from build123d import *

# Parameters (mm, degrees)
SKETCH1_R           = 14.2875
BOSS_EXTRUDE1_DEPTH = 3.175
CUT_EXTRUDE1_REACH  = 5.175
SKETCH2_R           = 2.667
CUT_EXTRUDE2_REACH  = 5.175
SKETCH4_R           = 6.35


with BuildPart() as part:
    # Sketch1 → Boss-Extrude1 (new body)
    with BuildSketch(Plane(origin=(0, 0, 0), x_dir=(1, 0, 0), z_dir=(0, 1, 0))):
        with BuildLine():
            Line((0, 25.4), (203.2, 25.4))
            ThreePointArc((203.2, 25.4), (228.6, 0), (203.2, -25.4))
            Line((203.2, -25.4), (0, -25.4))
            ThreePointArc((0, -25.4), (-25.4, 0), (0, 25.4))
        make_face()
        Circle(SKETCH1_R, mode=Mode.SUBTRACT)
        with Locations((203.2, 0)):
            Circle(SKETCH1_R, mode=Mode.SUBTRACT)
    extrude(amount=BOSS_EXTRUDE1_DEPTH)

    # Sketch2 → Cut-Extrude1 (cut, up to next)
    with BuildSketch(Plane(origin=(0, 3.175, 0), x_dir=(1, 0, 0), z_dir=(0, 1, 0)), mode=Mode.PRIVATE) as cut_extrude1_sk1:
        with Locations((101.6, 0)):
            Circle(SKETCH2_R)
    cut_extrude1_tool1 = extrude(cut_extrude1_sk1.sketch, amount=-CUT_EXTRUDE1_REACH, mode=Mode.PRIVATE) & part.part
    add(cut_extrude1_tool1.solids().sort_by_distance((101.6, 3.175, 0))[0], mode=Mode.SUBTRACT)

    # Sketch4 → Cut-Extrude2 (cut, up to next)
    with BuildSketch(Plane.XZ, mode=Mode.PRIVATE) as cut_extrude2_sk1:
        with Locations((30.1625, -12.7)):
            Circle(SKETCH4_R)
    cut_extrude2_tool1 = extrude(cut_extrude2_sk1.sketch, amount=-CUT_EXTRUDE2_REACH, mode=Mode.PRIVATE) & part.part
    add(cut_extrude2_tool1.solids().sort_by_distance((30.1625, 0, -12.7))[0], mode=Mode.SUBTRACT)
    # Sketch4 → Cut-Extrude2 (cut, up to next)
    with BuildSketch(Plane.XZ, mode=Mode.PRIVATE) as cut_extrude2_sk2:
        with Locations((49.2125, -12.7)):
            Circle(SKETCH4_R)
    cut_extrude2_tool2 = extrude(cut_extrude2_sk2.sketch, amount=-CUT_EXTRUDE2_REACH, mode=Mode.PRIVATE) & part.part
    add(cut_extrude2_tool2.solids().sort_by_distance((49.2125, 0, -12.7))[0], mode=Mode.SUBTRACT)
    # Sketch4 → Cut-Extrude2 (cut, up to next)
    with BuildSketch(Plane.XZ, mode=Mode.PRIVATE) as cut_extrude2_sk3:
        with Locations((68.2625, -12.7)):
            Circle(SKETCH4_R)
    cut_extrude2_tool3 = extrude(cut_extrude2_sk3.sketch, amount=-CUT_EXTRUDE2_REACH, mode=Mode.PRIVATE) & part.part
    add(cut_extrude2_tool3.solids().sort_by_distance((68.2625, 0, -12.7))[0], mode=Mode.SUBTRACT)
    # Sketch4 → Cut-Extrude2 (cut, up to next)
    with BuildSketch(Plane.XZ, mode=Mode.PRIVATE) as cut_extrude2_sk4:
        with Locations((87.3125, -12.7)):
            Circle(SKETCH4_R)
    cut_extrude2_tool4 = extrude(cut_extrude2_sk4.sketch, amount=-CUT_EXTRUDE2_REACH, mode=Mode.PRIVATE) & part.part
    add(cut_extrude2_tool4.solids().sort_by_distance((87.3125, 0, -12.7))[0], mode=Mode.SUBTRACT)
    # Sketch4 → Cut-Extrude2 (cut, up to next)
    with BuildSketch(Plane.XZ, mode=Mode.PRIVATE) as cut_extrude2_sk5:
        with Locations((106.3625, -12.7)):
            Circle(SKETCH4_R)
    cut_extrude2_tool5 = extrude(cut_extrude2_sk5.sketch, amount=-CUT_EXTRUDE2_REACH, mode=Mode.PRIVATE) & part.part
    add(cut_extrude2_tool5.solids().sort_by_distance((106.3625, 0, -12.7))[0], mode=Mode.SUBTRACT)
    # Sketch4 → Cut-Extrude2 (cut, up to next)
    with BuildSketch(Plane.XZ, mode=Mode.PRIVATE) as cut_extrude2_sk6:
        with Locations((125.4125, -12.7)):
            Circle(SKETCH4_R)
    cut_extrude2_tool6 = extrude(cut_extrude2_sk6.sketch, amount=-CUT_EXTRUDE2_REACH, mode=Mode.PRIVATE) & part.part
    add(cut_extrude2_tool6.solids().sort_by_distance((125.4125, 0, -12.7))[0], mode=Mode.SUBTRACT)
    # Sketch4 → Cut-Extrude2 (cut, up to next)
    with BuildSketch(Plane.XZ, mode=Mode.PRIVATE) as cut_extrude2_sk7:
        with Locations((144.4625, -12.7)):
            Circle(SKETCH4_R)
    cut_extrude2_tool7 = extrude(cut_extrude2_sk7.sketch, amount=-CUT_EXTRUDE2_REACH, mode=Mode.PRIVATE) & part.part
    add(cut_extrude2_tool7.solids().sort_by_distance((144.4625, 0, -12.7))[0], mode=Mode.SUBTRACT)
    # Sketch4 → Cut-Extrude2 (cut, up to next)
    with BuildSketch(Plane.XZ, mode=Mode.PRIVATE) as cut_extrude2_sk8:
        with Locations((163.5125, -12.7)):
            Circle(SKETCH4_R)
    cut_extrude2_tool8 = extrude(cut_extrude2_sk8.sketch, amount=-CUT_EXTRUDE2_REACH, mode=Mode.PRIVATE) & part.part
    add(cut_extrude2_tool8.solids().sort_by_distance((163.5125, 0, -12.7))[0], mode=Mode.SUBTRACT)
    # Sketch4 → Cut-Extrude2 (cut, up to next)
    with BuildSketch(Plane.XZ, mode=Mode.PRIVATE) as cut_extrude2_sk9:
        with Locations((39.6875, 12.7)):
            Circle(SKETCH4_R)
    cut_extrude2_tool9 = extrude(cut_extrude2_sk9.sketch, amount=-CUT_EXTRUDE2_REACH, mode=Mode.PRIVATE) & part.part
    add(cut_extrude2_tool9.solids().sort_by_distance((39.6875, 0, 12.7))[0], mode=Mode.SUBTRACT)
    # Sketch4 → Cut-Extrude2 (cut, up to next)
    with BuildSketch(Plane.XZ, mode=Mode.PRIVATE) as cut_extrude2_sk10:
        with Locations((58.7375, 12.7)):
            Circle(SKETCH4_R)
    cut_extrude2_tool10 = extrude(cut_extrude2_sk10.sketch, amount=-CUT_EXTRUDE2_REACH, mode=Mode.PRIVATE) & part.part
    add(cut_extrude2_tool10.solids().sort_by_distance((58.7375, 0, 12.7))[0], mode=Mode.SUBTRACT)
    # Sketch4 → Cut-Extrude2 (cut, up to next)
    with BuildSketch(Plane.XZ, mode=Mode.PRIVATE) as cut_extrude2_sk11:
        with Locations((77.7875, 12.7)):
            Circle(SKETCH4_R)
    cut_extrude2_tool11 = extrude(cut_extrude2_sk11.sketch, amount=-CUT_EXTRUDE2_REACH, mode=Mode.PRIVATE) & part.part
    add(cut_extrude2_tool11.solids().sort_by_distance((77.7875, 0, 12.7))[0], mode=Mode.SUBTRACT)
    # Sketch4 → Cut-Extrude2 (cut, up to next)
    with BuildSketch(Plane.XZ, mode=Mode.PRIVATE) as cut_extrude2_sk12:
        with Locations((96.8375, 12.7)):
            Circle(SKETCH4_R)
    cut_extrude2_tool12 = extrude(cut_extrude2_sk12.sketch, amount=-CUT_EXTRUDE2_REACH, mode=Mode.PRIVATE) & part.part
    add(cut_extrude2_tool12.solids().sort_by_distance((96.8375, 0, 12.7))[0], mode=Mode.SUBTRACT)
    # Sketch4 → Cut-Extrude2 (cut, up to next)
    with BuildSketch(Plane.XZ, mode=Mode.PRIVATE) as cut_extrude2_sk13:
        with Locations((115.8875, 12.7)):
            Circle(SKETCH4_R)
    cut_extrude2_tool13 = extrude(cut_extrude2_sk13.sketch, amount=-CUT_EXTRUDE2_REACH, mode=Mode.PRIVATE) & part.part
    add(cut_extrude2_tool13.solids().sort_by_distance((115.8875, 0, 12.7))[0], mode=Mode.SUBTRACT)
    # Sketch4 → Cut-Extrude2 (cut, up to next)
    with BuildSketch(Plane.XZ, mode=Mode.PRIVATE) as cut_extrude2_sk14:
        with Locations((134.9375, 12.7)):
            Circle(SKETCH4_R)
    cut_extrude2_tool14 = extrude(cut_extrude2_sk14.sketch, amount=-CUT_EXTRUDE2_REACH, mode=Mode.PRIVATE) & part.part
    add(cut_extrude2_tool14.solids().sort_by_distance((134.9375, 0, 12.7))[0], mode=Mode.SUBTRACT)
    # Sketch4 → Cut-Extrude2 (cut, up to next)
    with BuildSketch(Plane.XZ, mode=Mode.PRIVATE) as cut_extrude2_sk15:
        with Locations((153.9875, 12.7)):
            Circle(SKETCH4_R)
    cut_extrude2_tool15 = extrude(cut_extrude2_sk15.sketch, amount=-CUT_EXTRUDE2_REACH, mode=Mode.PRIVATE) & part.part
    add(cut_extrude2_tool15.solids().sort_by_distance((153.9875, 0, 12.7))[0], mode=Mode.SUBTRACT)
    # Sketch4 → Cut-Extrude2 (cut, up to next)
    with BuildSketch(Plane.XZ, mode=Mode.PRIVATE) as cut_extrude2_sk16:
        with Locations((173.0375, 12.7)):
            Circle(SKETCH4_R)
    cut_extrude2_tool16 = extrude(cut_extrude2_sk16.sketch, amount=-CUT_EXTRUDE2_REACH, mode=Mode.PRIVATE) & part.part
    add(cut_extrude2_tool16.solids().sort_by_distance((173.0375, 0, 12.7))[0], mode=Mode.SUBTRACT)


solid = part.part
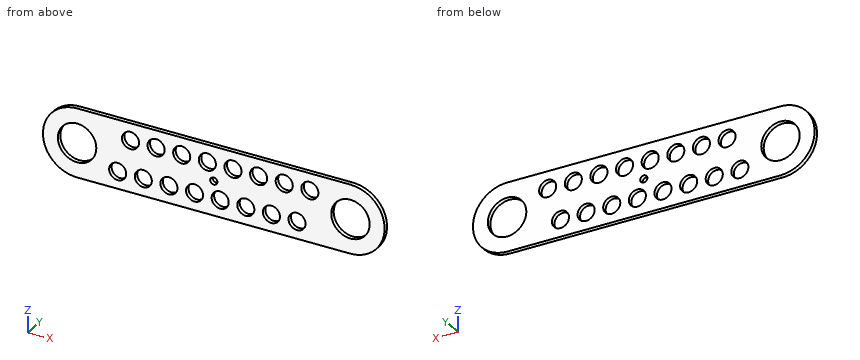
Here's how the part is built. I have some questions about the finished solid (model axes, mm). Give positions to 0.01 mm unless a question says otherwise; leave off trailing zeros. Order: outer loops, then holes, each group sorted by start corner. A loop starts at its lowest first (then second) coordinate and runs counter-clockwise, first axis right, second up. Notation, with made-up numbers: M 8.25,-15 L 50.25,-15 A28 cw 50.25,4 Z; hole C -19.5,-35.75 d6. An arc over 180 degrees is marked long. Answer as a JSON object with one key per item and string values. Group by question number.
1) Suppose I cut it at B-B, the plane y = 0.5. Count the separate pieces of the cut face and the enclosed holes in it, plus the area to 3 significant figures.
2) Please list where these lines run through material, in increasing order: L1, parallel to X at y = 2.2, z = 0; L2, parallel to Z at x = 111.5, y = 1.1; L3, parallel to Z at x = 68, y = 3. Write a range as [from, to].
3) Suppose I cut it at A-A, the plane z = 0. Write out the boundary of the cut face in (x, y) (1 decimal).
4) Suppose I cut it at C-C, the plane x = 116.5. Write out the boundary of the cut face in (y, z) (3 decimals), plus the area to 3 significant figures.
5) I'm going to push a flat-ended pin straight in: pin 1 Ø1 at (y, z) = (1, -6) entering from +X. Where does the tip first touch, or does it pass through?
Results found:
{
 "1": {"separate pieces": "1", "enclosed holes": "19", "area": "9,020 mm²"},
 "2": {"L1": "[-25.4, -14.29], [14.29, 98.93], [104.27, 188.91], [217.49, 228.6]", "L2": "[-25.4, -16.43], [-8.97, 8.11], [17.29, 25.4]", "L3": "[-25.4, -19.04], [-6.36, 25.4]"},
 "3": {"outline": "M -25.4,0 L -14.3,0 L -14.3,3.2 L -25.4,3.2 Z; M 14.3,0 L 98.9,0 L 98.9,3.2 L 14.3,3.2 Z; M 104.3,0 L 188.9,0 L 188.9,3.2 L 104.3,3.2 Z; M 217.5,0 L 228.6,0 L 228.6,3.2 L 217.5,3.2 Z"},
 "4": {"outline": "M 0,-25.4 L 3.175,-25.4 L 3.175,6.38 L 0,6.38 Z; M 0,19.02 L 3.175,19.02 L 3.175,25.4 L 0,25.4 Z", "area": "121 mm²"},
 "5": {"pin 1": "x = 228"}
}
